Verification items for this drawing (mm, ordinates from the low corner). A direction names the side the tool comes from. Coordinates: 2 decimals unless noted, no trailing zeros. Write each loop counter-clockwise with the first axis right and the second up, starting at its lowest first coordinate (ties: lowest second). Pieces come first, ordered by that corner, then holes.
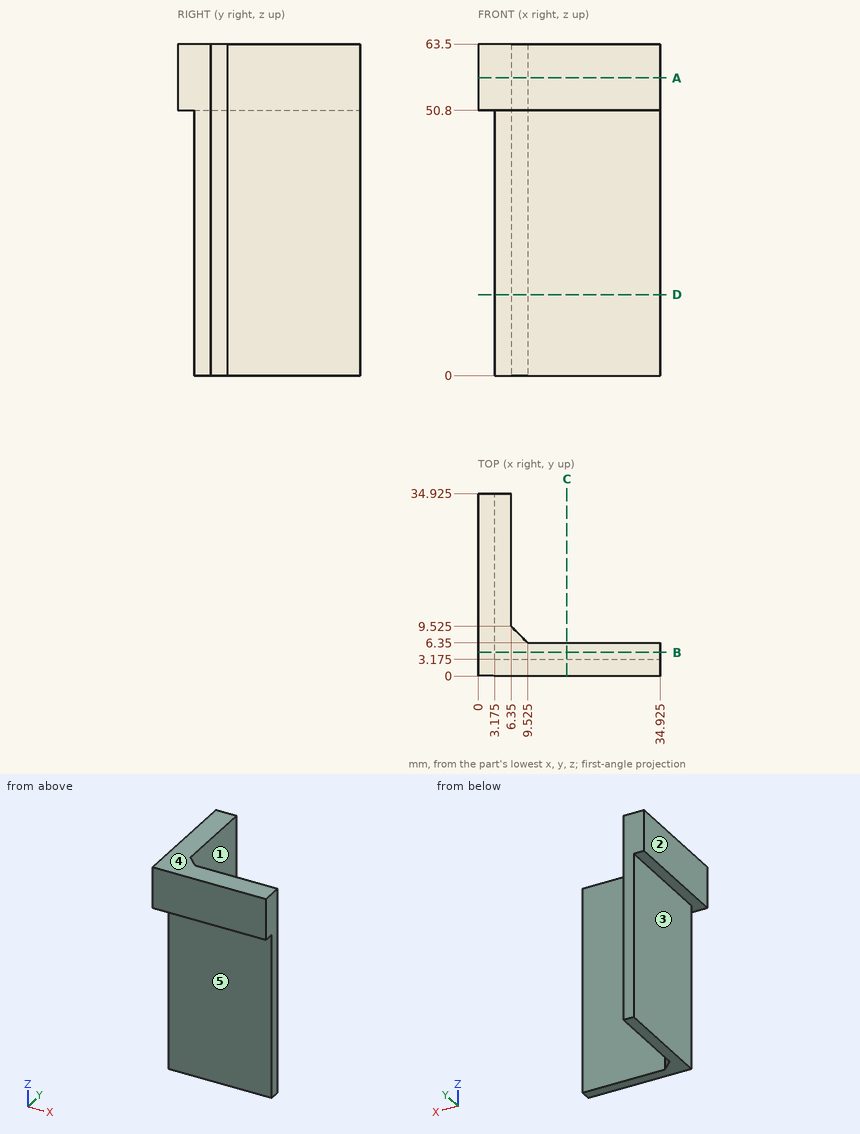
1. Sectioned sample at C-C, the plane x = 17. Record the boundary of the cut face in (y, z) (3 decimals).
Computed values:
outline: (0, 50.8) - (3.175, 50.8) - (3.175, 0) - (6.35, 0) - (6.35, 63.5) - (0, 63.5) - close
2. Sectioned sample at A-A, the plane z = 57. Record the boundary of the cut face in (x, y) (3 decimals).
Computed values:
outline: (0, 0) - (34.925, 0) - (34.925, 6.35) - (9.525, 6.35) - (6.35, 9.525) - (6.35, 34.925) - (0, 34.925) - close
3. Access from +Z, -Z, +X, -X, +Y, -Y to the whole of each face (thin tool, end or side, straight path). Record for the marked faces 1, 2, 3, 4 and 5.
Computed values:
face 1: +Z, -Z, +X, +Y
face 2: +Z, -Z, -X, +Y, -Y
face 3: -Z, -X, +Y, -Y
face 4: +Z, +X, -X, +Y, -Y
face 5: -Z, +X, -X, -Y
4. Sectioned sample at D-D, the plane z = 15.5. Record the boundary of the cut face in (x, y) (3 decimals), and give its area (3 significant figures).
Computed values:
outline: (3.175, 3.175) - (34.925, 3.175) - (34.925, 6.35) - (9.525, 6.35) - (6.35, 9.525) - (6.35, 34.925) - (3.175, 34.925) - close
area: 197 mm2
5. Sectioned sample at B-B, the plane y = 4.5. Record the boundary of the cut face in (x, z) (3 decimals).
Computed values:
outline: (0, 50.8) - (3.175, 50.8) - (3.175, 0) - (34.925, 0) - (34.925, 63.5) - (0, 63.5) - close
6. Thickness scan on line 1 along Y through (x, z) = (27, 48) (3 decimals); line 2 along X through (y, z) = (3.5, 37) (3 decimals). Record the ranges inside material, lowest first.
Computed values:
line 1: y = 3.175 to 6.35
line 2: x = 3.175 to 34.925
7. Gauge pin test, flat ends, axial feed: pin 1 Ø3 at (y, z) = (22, 31) entering from -X (3 decimals); pin 2 Ø12.5 at (y, z) = (25.5, 41.5) entering from +X; pin 3 Ø12.5 at (x, z) = (28, 23) entering from +Y; pin 4 Ø2 at (x, y) = (12, 6.5) entering from -Z. Record the tip position at first contact, or that the pin passes through.
Computed values:
pin 1: stops at x = 3.175
pin 2: stops at x = 6.35
pin 3: stops at y = 6.35
pin 4: stops at z = 0
